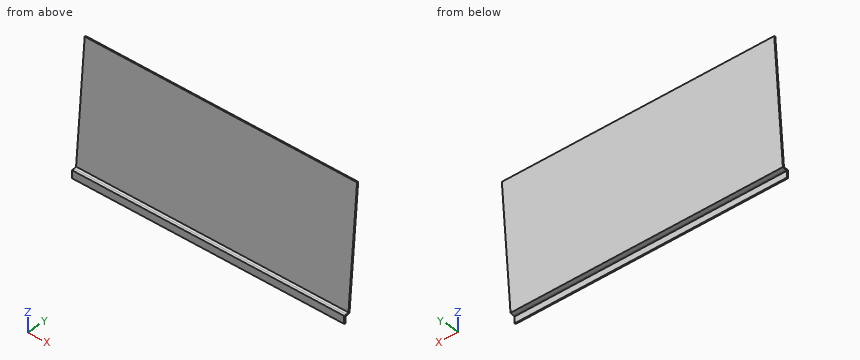
Autodesk Inventor part; units mm, degrees
ref_plane "YZ Plane" through (0, 0, 0) normal (1, 0, 0) x (0, 1, 0)
ref_plane "XZ Plane" through (0, 0, 0) normal (0, 1, 0) x (-1, 0, 0)
ref_plane "XY Plane" through (0, 0, 0) normal (0, 0, 1) x (1, 0, 0)
sketch "Sketch1" plane through (0, 0, 0) normal (1, 0, 0) x (0, 1, 0)
  line L0 (0, 0) -> (0, 597.7382)
  line L1 (0, 0) -> (3.175, 0)
  line L2 (3.175, 0) -> (3.175, 594.5632)
  line L3 (3.175, 594.5632) -> (9.906, 594.5632)
  line L4 (9.906, 594.5632) -> (15.756, 595.9828)
  line L5 (0, 597.7382) -> (9.5263, 597.7382)
  line L6 (9.5263, 597.7382) -> (12.7824, 598.5283)
  line L7 (41.2921, 902.0052) -> (15.756, 595.9828)
  line L8 (12.7824, 598.5283) -> (38.1281, 902.2692)
  line L9 (38.1281, 902.2692) -> (41.2921, 902.0052)
  line L10 (41.2921, 902.0052) -> (44.4671, 901.7403)
  line L11 (44.4671, 901.7403) -> (18.7409, 593.44)
  line L12 (18.7409, 593.44) -> (10.2857, 591.3882)
  line L13 (10.2857, 591.3882) -> (6.35, 591.3882)
  line L14 (6.35, 591.3882) -> (6.35, 574.5988)
  line L15 (6.35, 574.5988) -> (3.175, 574.5988)
  dimension "d0" = 594.5632
  dimension "d1" = 3.175
  dimension "d2" = 6.731
  dimension "d7" = 3.175
  dimension "d8" = 6.0198
  dimension "d9" = 166.36
  dimension "d10" = 3.175
  dimension "d11" = 108.41
  dimension "d12" = 3.175
  dimension "d13" = 307.086
  dimension "d16" = 3.175
  dimension "d18" = 3.175
  dimension "d20" = 307.1025
  dimension "d21" = 8.7006
  dimension "d22" = 3.175
  dimension "d23" = 3.175
  dimension "d24" = 3.9357
  dimension "d25" = 16.7894
extrude "Extrusion2" add sketch "Sketch1" along normal blind 720.725 contours L2 L3 L4 L7 L10 L11 L12 L13 L14 L15
properties part number "First_Shingle_Over_Intake_Vent_With_Length_28.375_Inches"
Work out the finished part from the listing and answer in its coordinate system (mm). Give positions to 0.01 mm unless a question says otherwise; leave off trailing zeros. Write each loop counter-clockwise with the first axis right and the second up, starting at its lowest first coordinate (ties: lowest second). Pieces come first, ordered by that corner, then holes. Notation, with made-up numbers: (31.5, 69) -> (87.5, 69) arc R16 ccw to (87.5, 73) -> close; hole circle Ø10 at (-21.75, -24.5). An arc over 180 degrees is marked (long way). Write item = value, one per line.
Q1. Section C-C on z = 624.5 is taken. Determine the outline of the cut face in (x, y) (3 decimals).
Computed values:
outline = (0, 18.136) -> (720.725, 18.136) -> (720.725, 21.333) -> (0, 21.333) -> close
Q2. Flat-ended cylindrical pins translate along their axes: pin 1 Ø4 at (x, z) = (530, 749) entering from +Y; pin 2 Ø1 at (x, y) = (514, 16) entering from -Z; pin 3 Ø10 at (x, y) = (378, 16.5) entering from -Z; pin 4 Ø3 at (x, y) = (230.5, 40.5) entering from +Z. Find the tip coordinate at first contact, or state that the pin passes through.
Computed values:
pin_1 = 31.89
pin_2 = 592.65
pin_3 = 591.68
pin_4 = 902.01
Q3. Consider line 1 along Z through (x, y) = (647.5, 5); line 2 along Y through (x, z) = (619, 680.5); line 3 along Y through (x, z) = (497, 607). Determine where each line is inside the solid, lowest interval first.
Computed values:
line_1 = 574.6 to 594.56
line_2 = 22.81 to 26.01
line_3 = 16.68 to 19.87
Q4. Section B-B on y = 35 is taken. Determine the outline of the cut face in (x, z) (3 decimals).
Computed values:
outline = (0, 788.287) -> (720.725, 788.287) -> (720.725, 826.601) -> (0, 826.601) -> close
Q5. Section A-A on x = 80 is taken. Determine the outline of the cut face in (y, z) (3 decimals).
Computed values:
outline = (3.175, 574.599) -> (6.35, 574.599) -> (6.35, 591.388) -> (10.286, 591.388) -> (18.741, 593.44) -> (44.467, 901.74) -> (41.292, 902.005) -> (15.756, 595.983) -> (9.906, 594.563) -> (3.175, 594.563) -> close
